from build123d import *

# Parameters (mm, degrees)
BOSS_EXTRUDE1_DEPTH = 5
BOSS_EXTRUDE2_DEPTH = 10


with BuildPart() as part:
    # Sketch1 → Boss-Extrude1 (new body)
    with BuildSketch(Plane.XY):
        Polygon((75.131397208, 20.131397208), (20.131397208, -75.131397208), (158.695461814, -155.131397208), (213.695461814, -59.868602792), align=None)
    extrude(amount=BOSS_EXTRUDE1_DEPTH)

    # Sketch2 → Boss-Extrude2 (add)
    with BuildSketch(Plane.XY.offset(5)):
        Polygon((158.695461814, -155.131397208), (213.695461814, -59.868602792), (75.131397208, 20.131397208), (20.131397208, -75.131397208), align=None)
        Polygon((26.961524227, -73.301270189), (156.865334795, -148.301270189), (206.865334795, -61.698729811), (76.961524227, 13.301270189), align=None, mode=Mode.SUBTRACT)
    extrude(amount=BOSS_EXTRUDE2_DEPTH)


solid = part.part
Model file for the job. Use its own axes, mm. A direction names the side the tool comes from. Give positions to 0.01 mm unless a question says otherwise; leave off trailing zeros. Loops run counter-clockwise (first coordinate to the right, second up) from the corner with the lowest first, then second, coordinate; pieces in that order, holes last.
Item 1: Drop flat-ended pins along their axis: P1, Ø5, axis at x = 149, y = -44, coming from the +Z side; P2, Ø1.5, axis at x = 89, z = 6, coming from the +Y side; P3, Ø8, axis at y = -44.5, z = 7, coming from the -X side. Give the stop position or say it passes through.
Check values:
P1: stops at z = 5
P2: stops at y = 12.56
P3: stops at x = 35.51
Item 2: Slice it at B-B (y = -49). Write the cut outline in (x, z), plus the area to 3 significant figures.
Check values:
outline: (35.22, 0) - (194.87, 0) - (194.87, 15) - (184.87, 15) - (184.87, 5) - (40.99, 5) - (40.99, 15) - (35.22, 15) - close
area: 956 mm2
Item 3: Which spindle directions (+Z, -Z, +X, -X, +Y, -Y) get a long thin tool onto all of the face, cutting with end or side? Do faces 5 (the face through (48.02, -26.83, 7.4)), 6 (the face through (91.004, -110.276, 9.93)). Say none if no direction does.
Check values:
face 5: +Z, -Z, -X, +Y
face 6: +Z
Item 4: Slice it at A-A (z = 11.5). Write the cut outline in (x, y).
Check values:
outline: (20.13, -75.13) - (158.7, -155.13) - (213.7, -59.87) - (75.13, 20.13) - close; hole (26.96, -73.3) - (156.87, -148.3) - (206.87, -61.7) - (76.96, 13.3) - close
Item 5: Slice it at C-C (x = 151). Write the cut outline in (y, z), plus the area to 3 significant figures.
Check values:
outline: (-150.69, 0) - (-23.67, 0) - (-23.67, 15) - (-29.44, 15) - (-29.44, 5) - (-144.91, 5) - (-144.91, 15) - (-150.69, 15) - close
area: 751 mm2
Item 6: Drill centre lines: line 1 along Z through (x, y) = (182, -75.5); line 2 along X through (y, z) = (-10, 8); line 3 along X through (y, z) = (6, 9.25). Where is each one in solid material? Low to high.
Check values:
line 1: z = 0 to 5
line 2: x = 57.74 to 63.51, 117.32 to 127.32
line 3: x = 66.97 to 72.75, 89.61 to 99.61
Item 7: Mould opens along Y. For faces 1 (the face through (185.81, -108.17, 7.4)), 2 (the face through (145.383, -20.429, 7.395)), 3 (the face through (52.312, -29.394, 9.93)), 4 (the face through (116, -66, 0)) say: +Y half, -Y half, draft (parallel to the pull), parting line (faces both ways), or undercut.
Check values:
face 1: -Y half
face 2: +Y half
face 3: undercut
face 4: draft
